Input: dimensioned drawing with shaded views. Units: mm. Origin: part minimum x, y, z. A direction names the side the tool comes from. Round coordinates to 2 decimals unless told otherwise and drop trailing zeros. Loops run counter-clockwise (first coordinate to the right, second up) from the corner with the lowest first, then second, coordinate; pieces in that order, holes last. Notation, with made-up numbers: (-19.5, -10.5) -> (33.5, -10.5) arc R22 ccw to (33.5, 16.5) -> close; hole circle Ø5 at (-20.75, -4). An arc over 180 degrees is marked (long way). Answer as a JSON object with one key per item and string values.
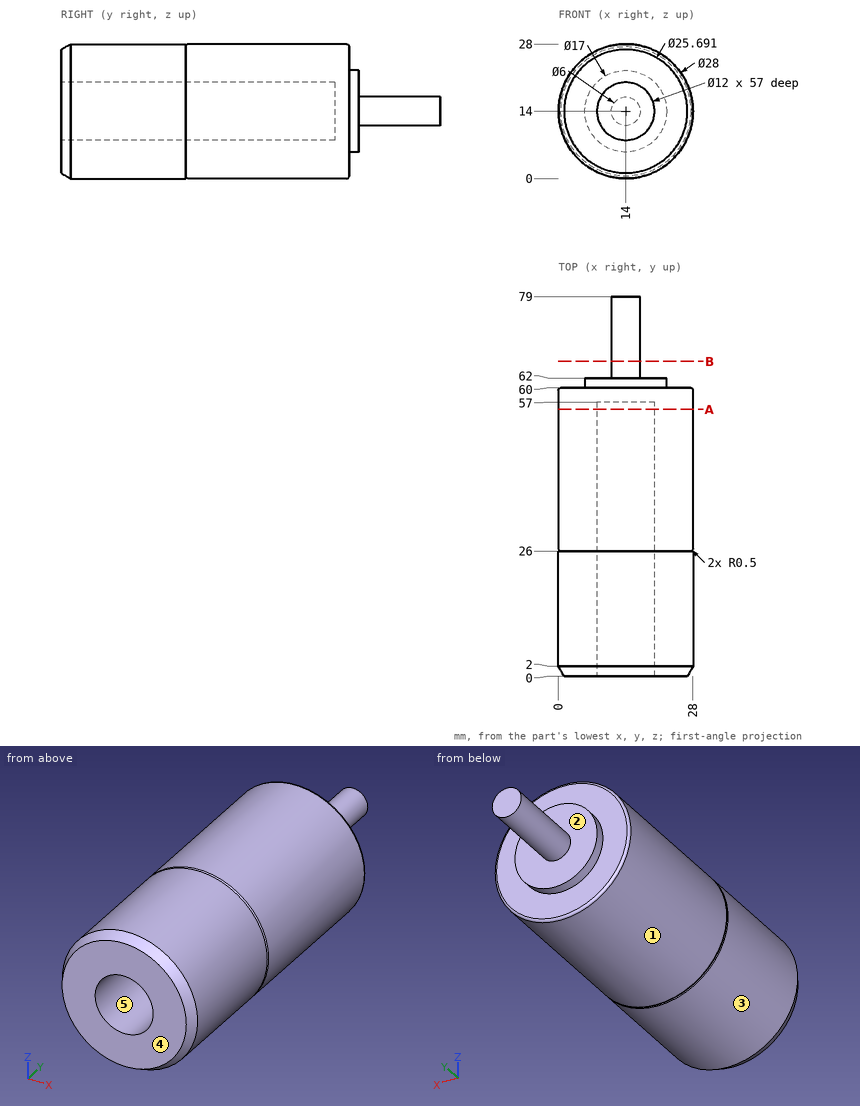
1) Reachability of the marked faces 1 and 2 from +Z, -Z, +X, -X, +Y, -Y: full face, straight path, thin tool, end or side. Return the list, or none.
Output:
{"face 1": "+Y, -Y", "face 2": "+Y"}
2) Section B-B, the plane y = 65.5. Output: boundary loops of the cut face in (x, z).
Output:
{"outline": "circle Ø6 at (14, 14)"}
3) Contact query for flat-ended pins moving along their axis: P1, Ø4, axis at x = 8.5, y = 41.5, coming from the +Z side (1 decimal); P2, Ø6, axis at x = 8.5, y = 9, coming from the -Z side (1 decimal); P3, Ø4, axis at x = 21.5, y = 51, coming from the +Z side (1 decimal). Output: stop coordinate, or through.
Output:
{"P1": "stops at z = 27.6", "P2": "stops at z = 0.2", "P3": "stops at z = 26.9"}
4) Section A-A, the plane y = 55.5. Output: boundary loops of the cut face in (x, z), plus the area to 3 significant figures.
Output:
{"outline": "circle Ø28 at (14, 14); hole circle Ø12 at (14, 14)", "area": "503 mm^2"}
5) Ray query, probe 1 along Z at (x, y) = (14, 28); probe 2 along Y at (x, z) = (23.5, 12.5); probe 3 along Z at (x, y) = (17.75, 12) (1 decimal). Return the intervals inside material, ascending.
Output:
{"probe 1": "z = 0 to 8, 20 to 28", "probe 2": "y = 0 to 60", "probe 3": "z = 0.5 to 9.3, 18.7 to 27.5"}
6) Draft query along X for the marked faces 3, 4 and 5. Return one class per face: +X half, -X half, draft (parallel to the pull), parting line (faces both ways), or undercut.
Output:
{"face 3": "parting line", "face 4": "draft", "face 5": "undercut"}
